Model file for the job. Use its own axes, mm. A direction names the side the tool comes from. Coordinates: 2 decimals unless noted, no trailing zeros. Loops run counter-clockwise (first coordinate to the right, second up) from the corner with the lowest first, then second, coordinate; pieces in that order, holes last.
from build123d import *

# Parameters (mm, degrees)
F0_W     = 43
F0_H     = 63
F1_DEPTH = 28
F2_R     = 9.9784830952
F3_DEPTH = 63
F4_T     = -1
F6_DEPTH = 47


with BuildPart() as f1:
    # F0 (on Top) → F1 (new body)
    with BuildSketch(Plane.XY):
        with Locations((26.4628629982, -6.1696139574)):
            Rectangle(F0_W, F0_H)
    extrude(amount=F1_DEPTH)

    # F2 (on face) → F3 (cut)
    with BuildSketch(Plane.XZ.offset(37.6696139574)):
        with Locations((26.4628629982, 16.9014558196)):
            Circle(F2_R)
    extrude(amount=-F3_DEPTH, mode=Mode.SUBTRACT)

    # F4
    f4_openings = [f1.faces().sort_by_distance(p)[0] for p in [
        (16.48438, -6.169614, 16.901456),
        (47.449735, 25.330386, 14),
    ]]
    offset(amount=F4_T, openings=f4_openings)

    # F5 (on face) → F6 (cut)
    with BuildSketch(Plane(origin=(0, 25.3303860426, 0), x_dir=(-1, 0, 0), z_dir=(0, 1, 0))):
        Polygon((-36.4628629982, 27), (-26.4628629982, 27), (-16.4644755423, 27), (-16.4644755423, 27.5), (-36.4628629982, 27.5), align=None)
    extrude(amount=-F6_DEPTH, mode=Mode.SUBTRACT)


solid = f1.part
Q1. Which spindle directions (+Z, -Z, +X, -X, +Y, -Y) get a long thin tool onto all of the face, cutting with end or side? Do faces 1 (the flat face through (46.963, -6, 14)), 2 (the flat face through (26.4, 25.33, 0.5)). Say none if no direction does.
Answers:
face 1: +Y
face 2: +Z, -Z, +X, -X, +Y
Q2. Slice it at B-B (z = 5.5). List the corners of the cut face in (x, y).
Answers:
outline: (4.96, -37.67) - (47.96, -37.67) - (47.96, 25.33) - (46.96, 25.33) - (46.96, -36.67) - (5.96, -36.67) - (5.96, 25.33) - (4.96, 25.33) - close
Q3. Flat gauge pins, fed straight in: P1, Ø16, axis at x = 26.46, z = 16.9, coming from the -Y side; P2, Ø5, axis at x = 15, z = 5, coming from the +Y side. Where does each tip first touch, or does it go through?
Answers:
P1: passes through
P2: stops at y = -36.67
Q4. Slice it at A-A (y = -22.5). List the corners of the cut face in (x, z), and give its area (3 significant figures).
Answers:
outline: (4.96, 0) - (47.96, 0) - (47.96, 28) - (4.96, 28) - close; hole (5.96, 1) - (46.96, 1) - (46.96, 27) - (5.96, 27) - close
area: 138 mm2
Q5. Slice it at C-C (x = 19.5). List the corners of the cut face in (y, z).
Answers:
outline: (-37.67, 0) - (25.33, 0) - (25.33, 1) - (-36.67, 1) - (-36.67, 9.75) - (-37.67, 9.75) - close; (-37.67, 24.05) - (-36.67, 24.05) - (-36.67, 27) - (-21.67, 27) - (-21.67, 27.5) - (25.33, 27.5) - (25.33, 28) - (-37.67, 28) - close
Q6. Slice it at D-D (z = 20.5). List the corners of the cut face in (x, y), and give its area (3 significant figures).
Answers:
outline: (4.96, -37.67) - (17.16, -37.67) - (17.16, -36.67) - (5.96, -36.67) - (5.96, 25.33) - (4.96, 25.33) - close; (35.77, -37.67) - (47.96, -37.67) - (47.96, 25.33) - (46.96, 25.33) - (46.96, -36.67) - (35.77, -36.67) - close
area: 148 mm2
Q7. Drill centre lines: line 1 (X direction, y = 21.5, z = 26.75); line 2 (Z direction, x = 16, y = 19.5); line 3 (Z direction, x = 35, y = -18.5). Where is each one in solid material? Low to high.
Answers:
line 1: x = 4.96 to 5.96, 46.96 to 47.96
line 2: z = 0 to 1, 27 to 28
line 3: z = 0 to 1, 27.5 to 28
Q8. Mould opens along X. For faces 3 (the flat face through (26, -6, 0)), 4 (the flat face through (21.6, -36.67, 8)), 5 (the flat face through (47.963, -7, 14)), 6 (the flat face through (4.963, -7, 14)) say: +X half, -X half, draft (parallel to the pull), parting line (faces both ways), or undercut.
Answers:
face 3: draft
face 4: undercut
face 5: +X half
face 6: -X half
